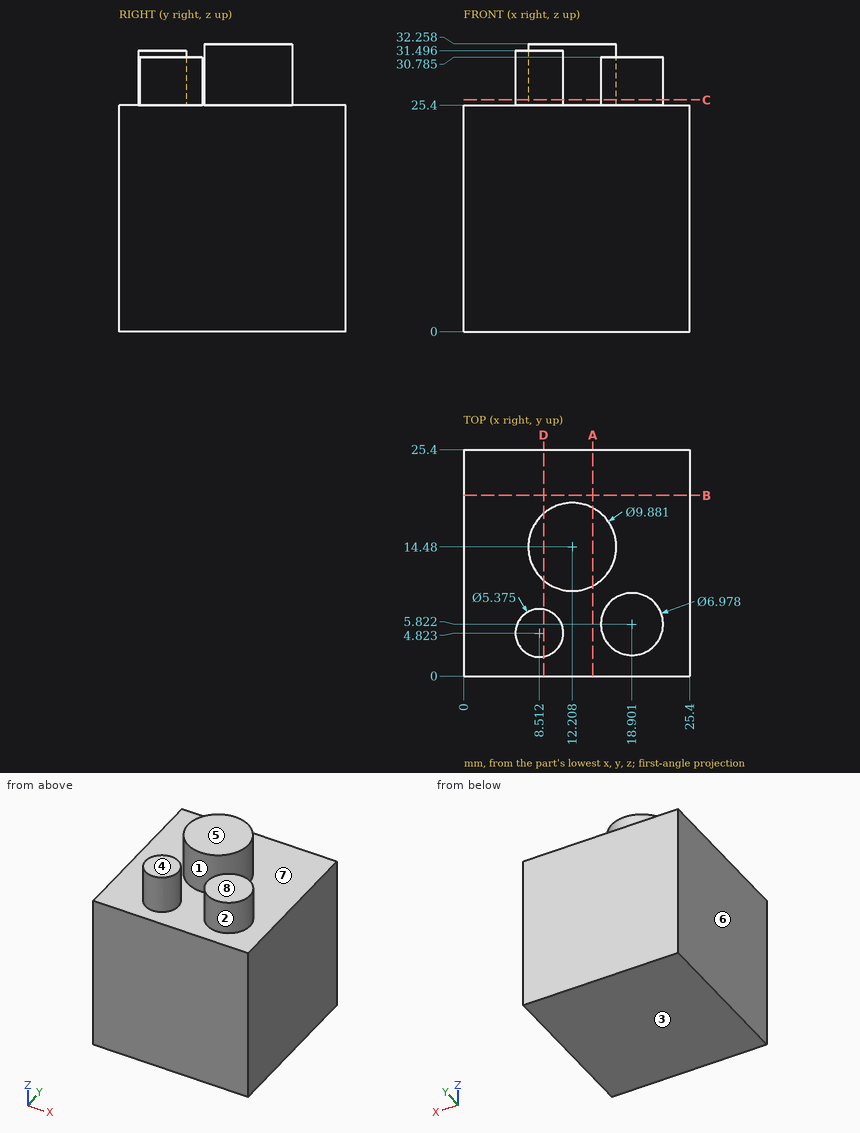
Drawing for the job (mm, zero at the part's lowest x, y, z). A direction names the side the tool comes from. Coordinates: 2 decimals unless noted, no trailing zeros. Order: outer loops, then holes, each group sorted by start corner. A loop starts at its lowest first (then second) coordinate and runs counter-clockwise, first axis right, second up. Notation, with made-up numbers: (-7, -29.5) - (45, -29.5) arc R27 cw to (45, -5.5) - close; hole circle Ø6 at (24.25, 88.5). An arc over 180 degrees is marked (long way). Use a Markdown table: item, result. Add a question column.
(1) Drill centre lines: line 1 along Z through (x, y) = (18.5, 11.25); line 2 along Z through (x, y) = (18, 3.75) (1 decimal). Where is each one in solid material? Low to high. Write a range as [from, to].
(2) Which spindle directions (+Z, -Z, +X, -X, +Y, -Y) get a long thin tool onto all of the face, cutting with end or side? Do the marked faces 4, 5, 6, 7 and 8. Say none if no direction does.
(3) Pull direction X, two halves, no side cores. Call the marked faces 1, 2 and 3: +X half, -X half, draft (parallel to the pull), parting line (faces both ways), or undercut.
(4) Flat gauge pins, fed straight in: pin 1 (3 mm diameter, centred on y = 16.5, z = 28, fed in from -X) (1 decimal); pin 2 (4 mm diameter, centred on x = 15.5, z = 19, fed in from -Y); pin 3 (4.5 mm diameter, centred on x = 8.5, y = 4.5, fed in from +Z); pin 4 (5.5 mm diameter, centred on x = 18, y = 7, fed in from +Z) (1 decimal). Where does each tip first touch, or does it go through?
(5) Saw through at D-D (x = 9). Give the cut face in (y, z), then the cut area to 3 significant figures.
(6) Saw through at A-A (x = 14.5). Give the cut face in (y, z).
(7) Saw through at C-C (z = 26). Give the cut face in (x, y) (1 decimal), then the cut area to 3 significant figures.
(8) Saw through at B-B (y = 20.25). Give the cut face in (x, z), then the cut area to 3 significant figures.
Solved:
| question | item | result |
|---|---|---|
| 1 | line 1 | z = [0, 25.4] |
| 1 | line 2 | z = [0, 30.8] |
| 2 | face 4 | +Z, +X, -X, -Y |
| 2 | face 5 | +Z, +X, -X, +Y, -Y |
| 2 | face 6 | +Z, -Z, -X, +Y, -Y |
| 2 | face 7 | +Z |
| 2 | face 8 | +Z, +X, -Y |
| 3 | face 1 | parting line |
| 3 | face 2 | undercut |
| 3 | face 3 | draft |
| 4 | pin 1 | stops at x = 7.3 |
| 4 | pin 2 | stops at y = 0 |
| 4 | pin 3 | stops at z = 31.5 |
| 4 | pin 4 | stops at z = 30.8 |
| 5 | outline | (0, 0) - (25.4, 0) - (25.4, 25.4) - (18.24, 25.4) - (18.24, 32.26) - (10.72, 32.26) - (10.72, 25.4) - (7.47, 25.4) - (7.47, 31.5) - (2.18, 31.5) - (2.18, 25.4) - (0, 25.4) - close |
| 5 | area | 729 mm² |
| 6 | outline | (0, 0) - (25.4, 0) - (25.4, 25.4) - (18.86, 25.4) - (18.86, 32.26) - (10.1, 32.26) - (10.1, 25.4) - (0, 25.4) - close |
| 7 | outline | circle Ø5.4 at (8.5, 4.8); circle Ø9.9 at (12.2, 14.5); circle Ø7 at (18.9, 5.8) |
| 7 | area | 138 mm² |
| 8 | outline | (0, 0) - (25.4, 0) - (25.4, 25.4) - (0, 25.4) - close |
| 8 | area | 645 mm² |
